```python
from build123d import *

# Parameters (mm, degrees)
F0_DEPTH = 2
F3_DEPTH = 5
F1_W     = 71
F1_H     = 29
F4_DEPTH = 7


with BuildPart() as f0:
    # F5 (on Top) → F0 (new body)
    with BuildSketch(Plane.XY):
        with BuildLine():
            Line((203.833783, 41.574535), (73.833783, 41.574535))
            ThreePointArc((73.833783, 41.574535), (43.833783, 4.074535), (73.833783, -33.425465))
            Line((73.833783, -33.425465), (203.833783, -33.425465))
            ThreePointArc((203.833783, -33.425465), (233.833783, 4.074535), (203.833783, 41.574535))
        make_face()
    extrude(amount=F0_DEPTH)

    # F2 (on face) → F3 (join)
    with BuildSketch(Plane.XY):
        with BuildLine():
            ThreePointArc((78.833783, 34.081681), (63.833783, 4.074535), (78.833783, -25.932611))
            Line((78.833783, -25.932611), (198.833783, -25.932611))
            ThreePointArc((198.833783, -25.932611), (213.833783, 4.074535), (198.833783, 34.081681))
            Line((198.833783, 34.081681), (78.833783, 34.081681))
        make_face()
    extrude(amount=-F3_DEPTH)

    # F1 (on face) → F4 (cut, through all)
    with BuildSketch(Plane.XY.offset(2)):
        with Locations((138.833783, 4.074535)):
            Rectangle(F1_W, F1_H)
    extrude(amount=-F4_DEPTH, mode=Mode.SUBTRACT)


solid = f0.part
```
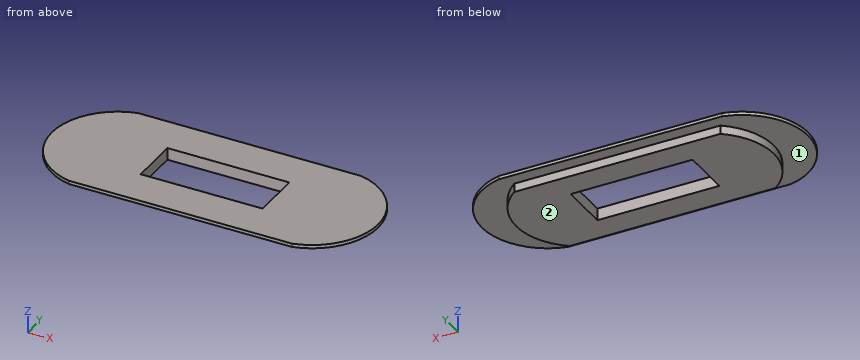
CAD build for the part. Positions are in the model's coordinates, mm. Face numbers are marked on the shaded views. A direction names the side the tool comes from. Round coordinates to 2 decimals unless told otherwise and drop trailing zeros. Order: outer loops, then holes, each group sorted by start corner. A loop starts at its lowest first (then second) coordinate and runs counter-clockwise, first axis right, second up.
Item 1: Saw through at C-C on y = 10.5. Write the cut outline in (x, z), then the cut area to 3 significant figures.
Item 2: Tool access for the marked faces 1 and 2: list every direction of +Z, -Z, +X, -X, +Y, -Y with a clear straight run to the whole face (end or side of a thin tool).
Item 3: Probe line 1 along X through (y, z) = (5, -0.75); line 2 along Y through (x, z) = (97.5, -0.75); line 3 along X through (y, z) = (-1, -4.25). List the from-to ranges inside material, lowest first.
Item 4: Saw through at D-D on x = 69. Write the cut outline in (y, z), then the cut area to 3 significant figures.
Item 5: Saw through at B-B on z = -2.5. Write the cut outline in (x, y).
Item 6: Saw through at A-A on x = 107.5. Write the cut outline in (y, z).
Item 7: Pin check, flat tips, straight feed: pin 1 (1.5 mm diameter, centred on x = 133.5, z = -3.5, fed in from -Y); pin 2 (1.5 mm diameter, centred on x = 112, z = -3, fed in from +Y). Stop position of each tip, or through.
Reported:
1. outline: (44.37, 0) - (64.39, 0) - (64.39, -5) - (103.33, -5) - (103.33, 2) - (44.37, 2) - close; (174.33, -5) - (213.28, -5) - (213.28, 0) - (233.29, 0) - (233.29, 2) - (174.33, 2) - close
1. area: 625 mm2
2. face 1: -Z
2. face 2: -Z, +X, -X, +Y, -Y
3. line 1: x = 63.85 to 103.33, 174.33 to 213.82
3. line 2: y = -25.93 to 34.08
3. line 3: x = 64.18 to 103.33, 174.33 to 213.49
4. outline: (-32, 0) - (-14.92, 0) - (-14.92, -5) - (23.07, -5) - (23.07, 0) - (40.15, 0) - (40.15, 2) - (-32, 2) - close
4. area: 334 mm2
5. outline: (78.83, -25.93) - (198.83, -25.93) arc R37.51 ccw to (198.83, 34.08) - (78.83, 34.08) arc R37.51 ccw to start; hole (103.33, -10.43) - (174.33, -10.43) - (174.33, 18.57) - (103.33, 18.57) - close
6. outline: (-33.43, 0) - (-25.93, 0) - (-25.93, -5) - (-10.43, -5) - (-10.43, 2) - (-33.43, 2) - close; (18.57, -5) - (34.08, -5) - (34.08, 0) - (41.57, 0) - (41.57, 2) - (18.57, 2) - close
7. pin 1: stops at y = -25.93
7. pin 2: stops at y = 34.08
